Design review of the part built by this model. Coordinates are the model's own, in mm. A direction names the side the tool comes from. Coordinates: 2 decimals unless noted, no trailing zeros. Loops run counter-clockwise (first coordinate to the right, second up) from the corner with the lowest first, then second, coordinate; pieces in that order, holes last. Notation, with made-up numbers: (-17, 39) - (-8, 39) arc R29 cw to (-8, 62) - close; hole circle Ø11 at (-2.5, 23). An arc over 180 degrees is marked (long way). Use one line per item in the form item = value. Start each with the question number.
(1) Add section A-A (x = 0). State the section outline as (y, z) points.
(2) Clearance check with flat-ended pins moving along their axes: pin 1 Ø1.5 at (x, z) = (-2.5, 2.5) entering from +Y; pin 2 Ø1 at (y, z) = (2.5, 5) entering from -X; pin 3 Ø1 at (x, z) = (3, 5.5) entering from -Y. State where each tip first meets the part, or that it passes through.
(3) For L1, parallel to Y at x = 0, z = 6.5; L2, parallel to Z at x = -0.75, y = 5.5; L3, parallel to X at y = 0.5, z = 2, list the stretches that pass through material, from the lowest coordinate up.
(4) The part is to be moulded in two halves that separate along X. For faces 3 (the face through (1.4, -1.4, 0)), 4 (the face through (0.37, 1.66, 4.31)), 5 (the face through (3.233, -1.341, 4.296)), say which applies: pulls with the +X half, pulls with the -X half, needs draft (parallel to the pull), parting line crosses it, or undercut.
(5) Add section C-C (z = 1.5). State the section outline as (x, y) points, plus the area to 3 significant figures.
(6) Add section D-D (y = -5.5). State the section outline as (x, z) points, plus the area to 3 significant figures.
(7) Tool access review of faces 1 (the face through (1.4, -1.4, 8.5)), 2 (the face through (3, -3, 1)): name each direction out of +Z, -Z, +X, -X, +Y, -Y from which nothing blocks a thin tool from reaching the whole face with its end or side.
```python
from build123d import *

# Parameters (mm, degrees)
F0_R     = 6.5
F0_R_2   = 3.5
F1_DEPTH = 1
F2_DEPTH = 4.25
F4_D     = 3.4


with BuildPart() as f1:
    # F0 (on Top) → F1 (new body)
    with BuildSketch(Plane.XY):
        Circle(F0_R)
        Circle(F0_R_2, mode=Mode.SUBTRACT)
        Circle(F0_R_2)
    extrude(amount=F1_DEPTH)

    # F0 (on Top) → F2 (join)
    with BuildSketch(Plane.XY):
        Circle(F0_R_2)
    extrude(amount=F2_DEPTH)

    # F3: F1 across face


with BuildPart() as f1_1:
    add(f1.part)
    add(f1.part.mirror(Plane.XY.offset(4.25)))

    # F4 (through all)
    with Locations(Plane(origin=(0, 0, 0), x_dir=(1, 0, 0), z_dir=(0, 0, -1))):
        with Locations((0, 0)):
            Hole(F4_D / 2)


solid = f1_1.part
```
Computed values:
q1.outline = (-6.5, 0) - (-1.7, 0) - (-1.7, 8.5) - (-6.5, 8.5) - (-6.5, 7.5) - (-3.5, 7.5) - (-3.5, 1) - (-6.5, 1) - close; (1.7, 0) - (6.5, 0) - (6.5, 1) - (3.5, 1) - (3.5, 7.5) - (6.5, 7.5) - (6.5, 8.5) - (1.7, 8.5) - close
q2.pin_1 = 3.03
q2.pin_2 = -2.87
q2.pin_3 = -2.45
q3.L1 = -3.5 to -1.7, 1.7 to 3.5
q3.L2 = 0 to 1, 7.5 to 8.5
q3.L3 = -3.46 to -1.62, 1.62 to 3.46
q4.face_3 = needs draft
q4.face_4 = undercut
q4.face_5 = parting line crosses it
q5.outline = circle Ø7 at (0, 0); hole circle Ø3.4 at (0, 0)
q5.area = 29.4 mm^2
q6.outline = (-3.46, 0) - (3.46, 0) - (3.46, 1) - (-3.46, 1) - close; (-3.46, 7.5) - (3.46, 7.5) - (3.46, 8.5) - (-3.46, 8.5) - close
q6.area = 13.9 mm^2
q7.face_1 = +Z, +X, -X, +Y, -Y
q7.face_2 = none
